from build123d import *

# Parameters (mm, degrees)
F0_W     = 150
F0_H     = 150
F1_DEPTH = 750
F2_SIZE  = 5
F3_R     = 45
F4_DEPTH = 50


with BuildPart() as f1:
    # F0 (on Front) → F1 (new body, symmetric)
    with BuildSketch(Plane.XZ):
        Rectangle(F0_W, F0_H)
    extrude(amount=F1_DEPTH, both=True)

    # F2
    f2_edges = [f1.edges().sort_by_distance(p)[0] for p in [
        (0, 750, 75),
        (-75, 0, 75),
        (0, -750, 75),
        (75, 0, 75),
    ]]
    chamfer(f2_edges, length=F2_SIZE)

    # F3 (on face) → F4 (cut)
    with BuildSketch(Plane.YZ.offset(75)):
        with Locations((-550, 0)):
            Circle(F3_R)
    extrude(amount=-F4_DEPTH, mode=Mode.SUBTRACT)


solid = f1.part
Geometry check sheet. Reference: the model listing, model coordinates, mm. A direction names the side the tool comes from. Round coordinates to 2 decimals unless told otherwise and drop trailing zeros. Loops run counter-clockwise (first coordinate to the right, second up) from the corner with the lowest first, then second, coordinate; pieces in that order, holes last. Notation, with made-up numbers: (39.5, 12.25) -> (43.5, 12.25) arc R30 cw to (43.5, 41.25) -> close; hole circle Ø8 at (29.5, -10.75). An arc over 180 degrees is marked (long way). Answer as a JSON object with one key per item and string values. Group by question number.
Item 1: Release check for a two-part mould opening along Z. For faces 1 (the face through (50.35, -507.08, 13.52)), 2 (the face through (-1, 750, -1)), 3 (the face through (-1, -10, -75)) record: pulls with the +Z half, pulls with the -Z half, needs draft (parallel to the pull), parting line crosses it, or undercut.
Item 2: Cross-section at B-B, the plane y = -550. Record the cut outline in (x, z).
Item 3: Cross-section at C-C, the plane z = 0. Record the cut outline in (x, y).
Item 4: Thickness scan on line 1 along Z through (x, y) = (38, -550); line 2 along X through (y, z) = (-542, -24.5); line 3 along Y through (x, z) = (62, -12). Record the ranges inside material, lowest first.
Item 5: Cross-section at A-A, the plane x = 49.5. Record the cut outline in (y, z).
Item 6: Set-up check for faces 4 (the face through (25, -551, 1)), 5 (the face through (-1, -750, -1)): record each of +Z, -Z, +X, -X, +Y, -Y from which the full face is reachable in a straight line by a thin tool's end or side.
Determined:
{
 "1": {"face 1": "undercut", "face 2": "needs draft", "face 3": "pulls with the -Z half"},
 "2": {"outline": "(-75, -75) -> (75, -75) -> (75, -45) -> (25, -45) -> (25, 45) -> (75, 45) -> (75, 70) -> (70, 75) -> (-70, 75) -> (-75, 70) -> close"},
 "3": {"outline": "(-75, -750) -> (75, -750) -> (75, -595) -> (25, -595) -> (25, -505) -> (75, -505) -> (75, 750) -> (-75, 750) -> close"},
 "4": {"line 1": "z = -75 to -45, 45 to 75", "line 2": "x = -75 to 25", "line 3": "y = -750 to -593.37, -506.63 to 750"},
 "5": {"outline": "(-750, -75) -> (750, -75) -> (750, 70) -> (745, 75) -> (-745, 75) -> (-750, 70) -> close; hole circle Ø90 at (-550, 0)"},
 "6": {"face 4": "+X", "face 5": "+Z, -Z, +X, -X, -Y"}
}
